Build history of the part. All positions in model axes, mm. Round coordinates to 2 decimals unless told otherwise and drop trailing zeros. Loops run counter-clockwise (first coordinate to the right, second up) from the corner with the lowest first, then second, coordinate; pieces in that order, holes last. Notation, with made-up numbers: (77.5, 86) -> (84.5, 86) arc R8 ccw to (84.5, 96) -> close; hole circle Ø7 at (49.25, 24). An arc over 180 degrees is marked (long way). Put each result on its own line as item: value. Start each with the question number.
Item 1: Cut at B-B, the plane z = 99. List the corners of the cut face in (x, y), plus the area to 3 significant figures.
Item 2: Flat gauge pins, fed straight in: pin 1 Ø1.7 at (x, z) = (-34.74, 63.5) entering from +Y; pin 2 Ø8 at (x, z) = (108.24, -160.84) entering from -Y; pin 3 Ø2 at (y, z) = (-5.5, 79.5) entering from +X. Where does each tip first touch, or does it go through?
Item 3: Cut at A-A, the plane y = -5. Count the separate pieces of the cut face and the enclosed holes in it, plus the area to 3 significant figures.
Item 4: Drill centre lines: probe 1 along Z at (x, y) = (166.5, -4.25); probe 2 along X at (y, z) = (-5, 63.5); probe 3 along Z at (x, y) = (70, -3.5). Where is each one in solid material? Low to high. Write a range as [from, to].
```python
from build123d import *

# Parameters (mm, degrees)
SKETCH1_W           = 313
SKETCH1_H           = 342
BOSS_EXTRUDE1_DEPTH = 6.35
SKETCH3_W           = 22
SKETCH3_H           = 155.14040353
SKETCH3_R           = 2.5
BOSS_EXTRUDE2_DEPTH = 6.35
SKETCH2_R           = 2.5
CUT_EXTRUDE1_DEPTH  = 7.35
SKETCH4_R           = 3.5
CUT_EXTRUDE2_DEPTH  = 7.35
CUT_EXTRUDE3_DEPTH  = 7.35
SKETCH6_R           = 1.5
CUT_EXTRUDE4_DEPTH  = 7.35
SKETCH7_R           = 1.05
CUT_EXTRUDE5_DEPTH  = 7.35


with BuildPart() as part:
    # Sketch1 → Boss-Extrude1 (new body)
    with BuildSketch(Plane(origin=(0, 0, 0), x_dir=(1, 0, 0), z_dir=(0, 1, 0))):
        Rectangle(SKETCH1_W, SKETCH1_H)
    extrude(amount=-BOSS_EXTRUDE1_DEPTH)

    # Sketch3 → Boss-Extrude2 (add)
    with BuildSketch(Plane(origin=(0, 0, 0), x_dir=(1, 0, 0), z_dir=(0, 1, 0))):
        with Locations((167.5, 9)):
            Rectangle(SKETCH3_W, SKETCH3_H)
        with Locations((166.5, 9)):
            Circle(SKETCH3_R, mode=Mode.SUBTRACT)
        with Locations((166.5, -41.8)):
            Circle(SKETCH3_R, mode=Mode.SUBTRACT)
        with Locations((166.5, 59.8)):
            Circle(SKETCH3_R, mode=Mode.SUBTRACT)
    extrude(amount=-BOSS_EXTRUDE2_DEPTH)

    # Sketch2 → Cut-Extrude1 (cut, through all)
    with BuildSketch(Plane(origin=(0, 0, 0), x_dir=(1, 0, 0), z_dir=(0, 1, 0))):
        with Locations((0, -123)):
            Circle(SKETCH2_R)
        with Locations((-70, -123)):
            Circle(SKETCH2_R)
        with Locations((70, -123)):
            Circle(SKETCH2_R)
        with Locations((-70, 141)):
            Circle(SKETCH2_R)
        with Locations((0, 141)):
            Circle(SKETCH2_R)
        with Locations((70, 141)):
            Circle(SKETCH2_R)
    extrude(amount=-CUT_EXTRUDE1_DEPTH, mode=Mode.SUBTRACT)

    # Sketch4 → Cut-Extrude2 (cut, through all)
    with BuildSketch(Plane(origin=(0, 0, 0), x_dir=(1, 0, 0), z_dir=(0, 1, 0))):
        with Locations((133.64, 160.84)):
            Circle(SKETCH4_R)
        with Locations((108.24, 160.84)):
            Circle(SKETCH4_R)
    cut_extrude2 = extrude(amount=-CUT_EXTRUDE2_DEPTH, mode=Mode.SUBTRACT)

    # Mirror1: Cut-Extrude2 across plane
    add(cut_extrude2.mirror(Plane(origin=(0, 0, -9), x_dir=(1, 0, 0), z_dir=(0, 0, -1))), mode=Mode.SUBTRACT)

    # Sketch5 → Cut-Extrude3 (cut, through all)
    with BuildSketch(Plane(origin=(0, 0, 0), x_dir=(1, 0, 0), z_dir=(0, 1, 0))):
        Polygon((139.671773243, 36.673783491), (147.171773243, 36.673783491), (147.143523721, -23.326216509), (139.643523721, -23.326216509), align=None)
    extrude(amount=-CUT_EXTRUDE3_DEPTH, mode=Mode.SUBTRACT)

    # Sketch6 → Cut-Extrude4 (cut, through all)
    with BuildSketch(Plane(origin=(0, 0, 0), x_dir=(1, 0, 0), z_dir=(0, 1, 0))):
        with Locations((60.32, 100.82)):
            Circle(SKETCH6_R)
        with Locations((10.32, 100.82)):
            Circle(SKETCH6_R)
        with Locations((10.32, -82.82)):
            Circle(SKETCH6_R)
        with Locations((60.32, -82.82)):
            Circle(SKETCH6_R)
    extrude(amount=-CUT_EXTRUDE4_DEPTH, mode=Mode.SUBTRACT)

    # Sketch7 → Cut-Extrude5 (cut, through all)
    with BuildSketch(Plane(origin=(0, 0, 0), x_dir=(1, 0, 0), z_dir=(0, 1, 0))):
        with Locations((-34.742947475, 81.5)):
            Circle(SKETCH7_R)
        with Locations((-34.742947475, -63.5)):
            Circle(SKETCH7_R)
        with Locations((-129.742947475, 81.5)):
            Circle(SKETCH7_R)
        with Locations((-129.742947475, -63.5)):
            Circle(SKETCH7_R)
        with Locations((108.411541633, 81.5)):
            Circle(SKETCH7_R)
        with Locations((108.411541633, -63.5)):
            Circle(SKETCH7_R)
        with Locations((24.439359852, 81.5)):
            Circle(SKETCH7_R)
        with Locations((24.439359852, -63.5)):
            Circle(SKETCH7_R)
    extrude(amount=-CUT_EXTRUDE5_DEPTH, mode=Mode.SUBTRACT)


solid = part.part
```
Reply:
1. outline: (-156.5, -6.35) -> (156.5, -6.35) -> (156.5, 0) -> (-156.5, 0) -> close
1. area: 1,990 mm^2
2. pin 1: passes through
2. pin 2: stops at y = -6.35
2. pin 3: stops at x = 156.5
3. separate pieces: 1
3. enclosed holes: 26
3. area: 110,000 mm^2
4. probe 1: z = [-86.57, -62.3], [-57.3, -11.5], [-6.5, 39.3], [44.3, 68.57]
4. probe 2: x = [-156.5, -130.79], [-128.69, -35.79], [-33.69, 23.39], [25.49, 107.36], [109.46, 178.5]
4. probe 3: z = [-171, -143.5], [-138.5, 120.5], [125.5, 171]
